Part model, mm, in its own coordinate system. A direction names the side the tool comes from. Give positions to 0.01 mm unless a question says otherwise; leave off trailing zeros. Write each loop counter-clockwise with the first axis right and the second up, starting at its lowest first coordinate (ties: lowest second). Pieces come first, ordered by that corner, then holes. Notation, with made-up numbers: M 46.25,55.25 L 56.25,55.25 A20 cw 56.25,79.25 Z; hole C 23.5,50.5 d8. An arc over 180 degrees is marked long. Use a Markdown table: item, result.
Autodesk Inventor part; units mm, degrees
ref_plane "ANBAU_XY" through (0, 0, -6) normal (0, 0, -1) x (1, 0, 0)
ref_plane "ANBAU_YZ" through (0, 0, -6) normal (1, 0, 0) x (0, -1, 0)
ref_plane "ANBAU_ZX" through (0, 0, -6) normal (0, -1, 0) x (0, 0, -1)
sketch "Skizze_1" plane through (0, 0, 0) normal (1, 0, 0) x (0, 1, 0)
  line L0 (0, -37.1) -> (0, 0)
  line L1 (0, 0) -> (5.7225, 0)
  line L2 (5.7225, 0) -> (6.5785, -0.856)
  line L3 (6.5785, -0.856) -> (6.5785, -6)
  line L4 (6.5785, -6) -> (8.5, -6)
  line L5 (8.5, -6) -> (8.5, -7.4)
  line L6 (8.5, -7.4) -> (10.2, -7.8555)
  line L7 (10.2, -7.8555) -> (10.2, -12.5445)
  line L8 (10.2, -12.5445) -> (8.5, -13)
  line L9 (8.5, -13) -> (5, -13)
  line L10 (5, -13) -> (5, -27.46)
  line L11 (5, -27.46) -> (5.5, -27.46)
  line L12 (5.5, -27.46) -> (5, -32.28)
  line L13 (5, -32.28) -> (5.5, -32.28)
  line L14 (5.5, -32.28) -> (5.0558, -36.5619)
  arc A0 (4.459, -37.1) -> (5.0558, -36.5619) centre (4.459, -36.5) ccw
  line L15 (4.459, -37.1) -> (0, -37.1)
  line L16 (0, -37.1) -> (0, 0)
revolve "Revolution1" add sketch "Skizze_1" angle 360 about axis through (0, 0, -37.1) along (0, 0, -1)
thread "Thread1"
sketch "Sketch2" plane through (0, 0, 0) normal (0, 0, 1) x (1, 0, 0)
  point P0 (0, 0)
hole "Hole1" at (0, 0, 0) direction (0, 0, -1) diameter 6.5 depth 37.1 countersink diameter 8.8094 countersink angle 60
sketch "Skizze_3" plane through (0, 0, 0) normal (0, 0, 1) x (1, 0, 0)
  line L0 (-17, -17) -> (17, -17)
  line L1 (17, -17) -> (17, 17)
  line L2 (17, 17) -> (-17, 17)
  line L3 (-17, 17) -> (-17, -17)
  line L4 (-8.5, -4.9075) -> (0, -9.815)
  line L5 (0, -9.815) -> (8.5, -4.9075)
  line L6 (8.5, -4.9075) -> (8.5, 4.9075)
  line L7 (8.5, 4.9075) -> (0, 9.815)
  line L8 (0, 9.815) -> (-8.5, 4.9075)
  line L9 (-8.5, 4.9075) -> (-8.5, -4.9075)
extrude "Extrusion1" cut sketch "Skizze_3" against normal blind 13
ref_plane "ANBAU_XY" through (0, 0, -6) normal (0, 0, -1) x (1, 0, 0)
ref_plane "ANBAU_YZ" through (0, 0, -6) normal (1, 0, 0) x (0, -1, 0)
ref_plane "ANBAU_ZX" through (0, 0, -6) normal (0, -1, 0) x (0, 0, -1)
ref_plane "ANBAU_STD_XY" through (0, 0, -6) normal (0, 0, -1) x (1, 0, 0)
ref_plane "ANBAU_STD_YZ" through (0, 0, -6) normal (1, 0, 0) x (0, -1, 0)
ref_plane "ANBAU_STD_ZX" through (0, 0, -6) normal (0, -1, 0) x (0, 0, -1)
properties part number "3607 N-1/4-P-9"
1. Two-plate mould, pull along Z, no slides. Class faces 1 (the cylindrical face through (-4.88, -1.08, -20.33)), 2 (the conical face through (5.107, -1.134, -34.867)), 3 (the flat face through (-4, 3, 0)), 4 (the flat face through (-8.5, 0, -10)): released by +Z, released by -Z, zero draft, split by the parting line, or undercut.
Findings below:
| item | result |
|---|---|
| face 1 | undercut |
| face 2 | released by -Z |
| face 3 | released by +Z |
| face 4 | zero draft |
2. Tool access for faces 5 (the conical face through (-0.229, -5.193, -30.372)), 6 (the cylindrical face through (7.167, 4.57, -6.71)), 7 (the conical face through (-0.19, -8.72, -12.94)): list every direction of +Z, -Z, +X, -X, +Y, -Y with a clear straight run to the whole face (end or side of a thin tool).
Findings below:
| item | result |
|---|---|
| face 5 | none |
| face 6 | +Z |
| face 7 | -Z, -Y |
3. Drop flat-ended pins along their axis: P1, Ø3.5, axis at x = -1.5, y = -0.5, coming from the +Z side; P2, Ø10, axis at y = -3.5, z = -25.5, coming from the -X side; P3, Ø6, axis at x = 4, z = -24, coming from the -Y side; P4, Ø6, axis at x = -4.5, y = -6, coming from the +Z side. Give the stop position or say it passes through.
Findings below:
| item | result |
|---|---|
| P1 | z = -1.86 |
| P2 | x = -5.5 |
| P3 | y = -4.9 |
| P4 | z = 0 |
4. Cut at C-C, the plane z = -18.5. Give the cut face in (x, y), then the cut area to 3 significant figures.
Findings below:
| item | result |
|---|---|
| outline | C 0,0 d10; hole C 0,0 d6.5 |
| area | 45.4 mm2 |
5. Drill centre lines: L1, parallel to X at y = 0, z = -12.5; L2, parallel to X at y = 0, z = -25; L3, parallel to Y at x = 0, z = -9 (3 decimals). Where is each one in solid material? Low to high.
Findings below:
| item | result |
|---|---|
| L1 | -8.5 to -3.25, 3.25 to 8.5 |
| L2 | -5 to -3.25, 3.25 to 5 |
| L3 | -9.815 to -3.25, 3.25 to 9.815 |
6. Cut at B-B, the plane z = -5.5. Give the cut face in (x, y), then the cut area to 3 significant figures.
Findings below:
| item | result |
|---|---|
| outline | C 0,0 d13.16; hole C 0,0 d6.5 |
| area | 103 mm2 |
